Geometry check sheet. Reference: the model listing, model coordinates, mm. Give positions to 0.01 mm unless a question says otherwise; leave off trailing zeros. Loops run counter-clockwise (first coordinate to the right, second up) from the corner with the lowest first, then second, coordinate; pieces in that order, holes last.
1. Go/stop test with flat-tipped pins: pin 1 Ø3 at (x, y) = (-3.5, 0.5) entering from +Z; pin 2 Ø1.5 at (x, y) = (-6.5, 2) entering from +Z; pin 3 Ø1.5 at (x, y) = (-4.5, 2.5) entering from +Z. Record where each tip stops, or that it passes through.
2. Material ranges on L1, parallel to X at y = 2.95, z = 9.5; L2, parallel to X at y = 3.85, z = 6.5; L3, parallel to Z at x = -1, y = 2.35, recorded low to high.
3. Cross-section at A-A, the plane y = 3.95. Record the cut outline in (x, z).
from build123d import *

# Parameters (mm, degrees)
BOSS_EXTRUDE1_DEPTH = 5
FILLET1_R           = 0.5


with BuildPart() as part:
    # Sketch1 → Boss-Extrude1 (new body)
    with BuildSketch(Plane(origin=(0, 0, 0), x_dir=(1, 0, 0), z_dir=(0, 1, 0))):
        with BuildLine():
            Line((-12.5, 0), (-20, 0))
            ThreePointArc((-20, 0), (-14.142135624, -14.142135624), (0, -20))
            Line((0, -20), (0, -12.5))
            ThreePointArc((0, -12.5), (-8.838834765, -8.838834765), (-12.5, 0))
        make_face()
    extrude(amount=BOSS_EXTRUDE1_DEPTH)

    # Fillet1
    fillet1_edges = [part.edges().sort_by_distance(p)[0] for p in [
        (-14.142135624, 5, 14.142135624),
        (0, 5, 16.25),
        (-8.838834765, 5, 8.838834765),
        (0, 0, 16.25),
        (-14.142135624, 0, 14.142135624),
        (-16.25, 0, 0),
        (-8.838834765, 0, 8.838834765),
        (0, 2.5, 12.5),
        (0, 2.5, 20),
        (-20, 2.5, 0),
        (-12.5, 2.5, 0),
        (-16.25, 5, 0),
    ]]
    fillet(fillet1_edges, radius=FILLET1_R)


solid = part.part
Result:
1. pin 1: stops at z = 19.9
1. pin 2: stops at z = 19.16
1. pin 3: stops at z = 19.65
2. L1: x = -17.6 to -8.12
2. L2: x = -18.91 to -10.68
2. L3: z = 12.46 to 19.97
3. outline: (-19.99, 0.51) arc R0.5 ccw to (-19.49, 0) - (-12.99, 0) arc R0.5 ccw to (-12.49, 0.48) arc R12.5 cw to (-0.48, 12.49) arc R0.5 ccw to (0, 12.99) - (0, 19.49) arc R0.5 ccw to (-0.51, 19.99) arc R20 ccw to start
